Here's how the part is built. I have some questions about the finished solid (model axes, mm). Face numbers are marked on the shaded views. A direction names the side the tool comes from. Coordinates: 2 decimals unless noted, no trailing zeros. Write each loop counter-clockwise with the first axis right and the second up, starting at its lowest first coordinate (ties: lowest second). Pieces come first, ordered by that corner, then holes. Notation, with made-up numbers: (50.25, 22.5) - (70.25, 22.5) arc R11 ccw to (70.25, 34.5) - close; hole circle Ø3 at (-27.75, 1). An arc over 180 degrees is marked (long way). Answer in a Markdown table with one row per item. Add a question column.
Item 1: Imagine slicing it at B-B (z = 23). Please give me the cut outline in (x, y).
Item 2: Which directions (+Z, -Z, +X, -X, +Y, -Y) give clear straight access to the entire face, cutting with the end or side of a thin tool? Please do the marked faces 4, 5, 6 and 7.
Item 3: I'm going to push flat-ended pins straight in: pin 1 (12 mm diameter, centred on x = -2.5, y = -13, fed in from -Z); pin 2 (2 mm diameter, centred on x = 0, z = 41.5, fed in from -Y); pin 3 (0.7 mm diameter, centred on x = 7.5, y = -27, fed in from +Z); pin 4 (10 mm diameter, centred on x = 2.5, z = 20, fed in from -Y). Where does each tip first touch, or does it pass through?
Item 4: If I drill on probe 1 along Y at (x, z) = (15.5, 38); probe 2 along Z at (x, y) = (-17, -14); probe 3 along Z at (x, y) = (-7.5, 2.5), over which ranges is the centre line in solid material (lowest first)? Write a range as from..to.
Item 5: Imagine slicing it at A-A (y = 0). Please give me the cut outline in (x, z).
Item 6: Imagine slicing it at D-D (x = -10). Please give me the cut outline in (y, z).
Item 7: Imagine slicing it at C-C (x = 0). Please give me the cut outline in (y, z).
Item 8: We'd pull the mould along Z, two halves only. Please class the marked faces 1, 2 and 3: +Z half, -Z half, draft (parallel to the pull), parting line (faces both ways), or undercut.
from build123d import *

# Parameters (mm, degrees)
SKETCH1_W           = 42
SKETCH1_H           = 42
BOSS_EXTRUDE1_DEPTH = 39
CHAMFER1_SIZE       = 5
SKETCH5_R           = 11
SKETCH5_R_2         = 2.5
BOSS_EXTRUDE2_DEPTH = 2
SKETCH6_R           = 2.5
BOSS_EXTRUDE3_DEPTH = 24
SKETCH7_W           = 5.502287021
SKETCH7_H           = 7.880652758
CUT_EXTRUDE1_DEPTH  = 15
SKETCH8_W           = 16
SKETCH8_H           = 13
BOSS_EXTRUDE4_DEPTH = 11
CUT_EXTRUDE2_START  = -8
SKETCH9_W           = 84.832687132
SKETCH9_H           = 82.051636753
CUT_EXTRUDE2_DEPTH  = 22


# Read off the part's stored shape, not the designer's step: M3x0.5 Tapped Hole1
with BuildPart() as part:
    # Sketch1 → Boss-Extrude1 (new body)
    with BuildSketch(Plane.XY):
        Rectangle(SKETCH1_W, SKETCH1_H)
    extrude(amount=BOSS_EXTRUDE1_DEPTH)

    # Chamfer1
    chamfer1_edges = [part.edges().sort_by_distance(p)[0] for p in [
        (21, -21, 19.5),
        (-21, -21, 19.5),
        (-21, 21, 19.5),
        (21, 21, 19.5),
    ]]
    chamfer(chamfer1_edges, length=CHAMFER1_SIZE)

    # M3x0.5 Tapped Hole1 outline → M3x0.5 Tapped Hole1 (revolve, cut)
    with BuildSketch(Plane(origin=(15.5, 15.5, 0), x_dir=(1, 0, 0), z_dir=(0, -1, 0))):
        Polygon((0, 39), (0, 33.748924226), (1.25, 34.5), (1.25, 39), align=None)
    revolve(axis=Axis((15.5, 15.5, 0), (0, 0, 1)), mode=Mode.SUBTRACT)

    # M3x0.5 Tapped Hole1 2 outline → M3x0.5 Tapped Hole1 2 (revolve, cut)
    with BuildSketch(Plane(origin=(-15.5, -15.5, 0), x_dir=(1, 0, 0), z_dir=(0, -1, 0))):
        Polygon((0, 39), (0, 33.748924226), (1.25, 34.5), (1.25, 39), align=None)
    revolve(axis=Axis((-15.5, -15.5, 0), (0, 0, 1)), mode=Mode.SUBTRACT)

    # M3x0.5 Tapped Hole1 3 outline → M3x0.5 Tapped Hole1 3 (revolve, cut)
    with BuildSketch(Plane(origin=(-15.5, 15.5, 0), x_dir=(1, 0, 0), z_dir=(0, -1, 0))):
        Polygon((0, 39), (0, 33.748924226), (1.25, 34.5), (1.25, 39), align=None)
    revolve(axis=Axis((-15.5, 15.5, 0), (0, 0, 1)), mode=Mode.SUBTRACT)

    # M3x0.5 Tapped Hole1 4 outline → M3x0.5 Tapped Hole1 4 (revolve, cut)
    with BuildSketch(Plane(origin=(15.5, -15.5, 0), x_dir=(1, 0, 0), z_dir=(0, -1, 0))):
        Polygon((0, 39), (0, 33.748924226), (1.25, 34.5), (1.25, 39), align=None)
    revolve(axis=Axis((15.5, -15.5, 0), (0, 0, 1)), mode=Mode.SUBTRACT)

    # Sketch5 → Boss-Extrude2 (add)
    with BuildSketch(Plane.XY.offset(39)):
        with Locations(Location((0, 0, 0), (0, 0, 180))):
            Circle(SKETCH5_R)
        Circle(SKETCH5_R_2, mode=Mode.SUBTRACT)
    extrude(amount=BOSS_EXTRUDE2_DEPTH)

    # Sketch6 → Boss-Extrude3 (add)
    with BuildSketch(Plane.XY.offset(39)):
        Circle(SKETCH6_R)
    extrude(amount=BOSS_EXTRUDE3_DEPTH)

    # Sketch7 → Cut-Extrude1 (cut)
    with BuildSketch(Plane.XY.offset(63)):
        with Locations((1.25114351, 5.940326379)):
            Rectangle(SKETCH7_W, SKETCH7_H)
    extrude(amount=-CUT_EXTRUDE1_DEPTH, mode=Mode.SUBTRACT)

    # Sketch8 → Boss-Extrude4 (add)
    with BuildSketch(Plane(origin=(0, 0, 0), x_dir=(-1, 0, 0), z_dir=(0, 0, -1))):
        with Locations((0, -21)):
            Rectangle(SKETCH8_W, SKETCH8_H)
    extrude(amount=-BOSS_EXTRUDE4_DEPTH)

    # Sketch9 → Cut-Extrude2 (cut)
    with BuildSketch(Plane.XY.offset(39).offset(CUT_EXTRUDE2_START)):
        with Locations((-5.67946535, 2.529712031)):
            Rectangle(SKETCH9_W, SKETCH9_H)
        Polygon((-34.171572875, 0), (0, 34.171572875), (34.171572875, 0), (0, -34.171572875), align=None, mode=Mode.SUBTRACT)
    extrude(amount=-CUT_EXTRUDE2_DEPTH, mode=Mode.SUBTRACT)


solid = part.part
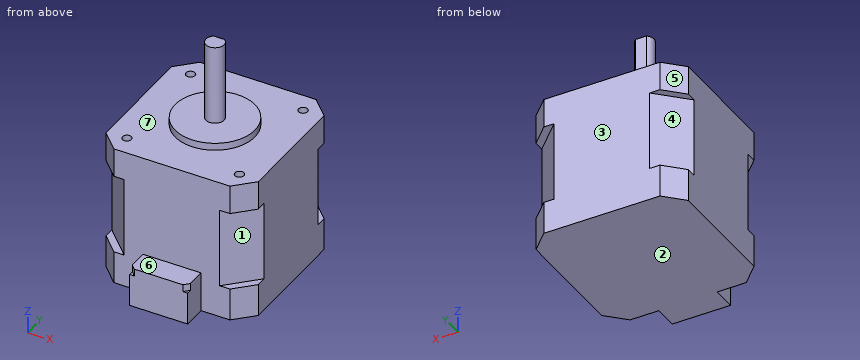
Here are the results:
| question | item | result |
|---|---|---|
| 1 | outline | (-21, -13.17) - (-13.17, -21) - (13.17, -21) - (21, -13.17) - (21, 13.17) - (13.17, 21) - (-13.17, 21) - (-21, 13.17) - close |
| 2 | face 4 | -X, +Y |
| 2 | face 5 | +Z, -Z, -X, +Y |
| 2 | face 6 | +Z, +X, -X, -Y |
| 2 | face 7 | +Z |
| 3 | pin 1 | stops at z = 0 |
| 3 | pin 2 | stops at y = -11 |
| 3 | pin 3 | stops at z = 11 |
| 3 | pin 4 | stops at y = -21 |
| 4 | probe 1 | y = -21..-16.75, -14.25..14.25, 16.75..21 |
| 4 | probe 2 | z = 0..39 |
| 4 | probe 3 | z = 0..41 |
| 5 | outline | (-21, 0) - (21, 0) - (21, 39) - (11, 39) - (11, 41) - (2.5, 41) - (2.5, 63) - (-2.5, 63) - (-2.5, 41) - (-11, 41) - (-11, 39) - (-21, 39) - close |
| 6 | outline | (-21, 0) - (21, 0) - (21, 39) - (4.58, 39) - (4.58, 41) - (-4.58, 41) - (-4.58, 39) - (-21, 39) - close |
| 7 | outline | (-27.5, 0) - (21, 0) - (21, 39) - (11, 39) - (11, 41) - (2.5, 41) - (2.5, 48) - (2, 48) - (2, 63) - (-2.5, 63) - (-2.5, 41) - (-11, 41) - (-11, 39) - (-21, 39) - (-21, 11) - (-27.5, 11) - close |
| 8 | face 1 | undercut |
| 8 | face 2 | -Z half |
| 8 | face 3 | draft |
